```python
from build123d import *

# Parameters (mm, degrees)
F1_DEPTH = 23
F2_W     = 55.3733881378
F2_H     = 29.1305183362
F3_DEPTH = 2


with BuildPart() as f1:
    # F0 (on Front) → F1 (new body)
    with BuildSketch(Plane.XZ):
        with BuildLine():
            Line((58.6916125421, -112.6401221338), (58.6916125421, -83.5096037976))
            ThreePointArc((58.6916125421, -83.5096037976), (63.4212285001, -31.2054716299), (12.2713760607, -19.2981585681))
            Line((12.2713760607, -19.2981585681), (12.2713760607, 27.3598778662))
            Line((12.2713760607, 27.3598778662), (0.550356732, 27.3598778662))
            Line((0.550356732, 27.3598778662), (0.550356732, -28.7071379409))
            ThreePointArc((0.550356732, -28.7071379409), (-8.9441612758, -56.657800803), (3.3182244043, -83.5096037976))
            Line((3.3182244043, -83.5096037976), (3.3182244043, -112.6401221338))
            Line((3.3182244043, -112.6401221338), (58.6916125421, -112.6401221338))
        make_face()
    extrude(amount=F1_DEPTH)

    # F2 (on face) → F3 (cut)
    with BuildSketch(Plane(origin=(0, 0, 0), x_dir=(-1, 0, 0), z_dir=(0, 1, 0))):
        with Locations((-31.0049184732, -98.0748629657)):
            Rectangle(F2_W, F2_H)
    extrude(amount=-F3_DEPTH, mode=Mode.SUBTRACT)


solid = f1.part
```
Model file for the job. Use its own axes, mm. A direction names the side the tool comes from. Coordinates: 2 decimals unless noted, no trailing zeros. Loops run counter-clockwise (first coordinate to the right, second up) from the corner with the lowest first, then second, coordinate; pieces in that order, holes last. Notation, with made-up numbers: (32, -28.5) - (67, -28.5) arc R13 cw to (67, -5.5) - close; hole circle Ø11 at (34.5, 79). An arc over 180 degrees is marked (long way). Answer as a JSON object with one key per item and string values. Group by question number.
(1) Flat gauge pins, fed straight in: pin 1 (1 mm diameter, centred on x = 27.5, y = -0.5, fed in from -Z); pin 2 (12 mm diameter, centred on y = -4.5, z = -74, fed in from +X); pin 3 (8 mm diameter, centred on x = 46, y = -6, fed in from +Z). Where does each tip first touch, or does it go through?
(2) Tool access for faces 1 (the face through (58.692, -12, -98)), 2 (the face through (0.55, -11, 0)), 3 (the face through (31, -2, -98)), 4 (the face through (6, -11, 27.36)), 5 (the face through (3.318, -12, -98)): list every direction of +Z, -Z, +X, -X, +Y, -Y with a clear straight run to the whole face (end or side of a thin tool).
(3) Probe line 1 along X through (y, z) = (-10, -97.5); line 2 along X through (y, z) = (-9.25, -7); line 3 along Y through (x, z) = (6, -95). List the from-to ranges inside material, lowest first.
(4) Cut at D-D (x = 22.5). Give the cut face in (y, z).
(5) Cut at A-A (y = -15.75). Give the cut face in (x, z).
(6) Cut at B-B (x = 8). Give the cut face in (y, z), then the cut area to 3 significant figures.
(7) Cut at C-C (z = -88). Give the cut face in (x, y).
Geometry says:
{
 "1": {"pin 1": "stops at z = -83.51", "pin 2": "stops at x = 68.71", "pin 3": "stops at z = -16.18"},
 "2": {"face 1": "-Z, +X, +Y, -Y", "face 2": "+Z, -X, +Y, -Y", "face 3": "-Z, +X, -X, +Y", "face 4": "+Z, +X, -X, +Y, -Y", "face 5": "-Z, -X, +Y, -Y"},
 "3": {"line 1": "x = 3.32 to 58.69", "line 2": "x = 0.55 to 12.27", "line 3": "y = -23 to -2"},
 "4": {"outline": "(-23, -112.64) - (-2, -112.64) - (-2, -83.51) - (0, -83.51) - (0, -15.55) - (-23, -15.55) - close"},
 "5": {"outline": "(0.55, -28.71) arc R40 ccw to (3.32, -83.51) - (3.32, -112.64) - (58.69, -112.64) - (58.69, -83.51) arc R40 ccw to (12.27, -19.3) - (12.27, 27.36) - (0.55, 27.36) - close"},
 "6": {"outline": "(-23, -112.64) - (-2, -112.64) - (-2, -83.51) - (0, -83.51) - (0, 27.36) - (-23, 27.36) - close", "area": "3,160 mm^2"},
 "7": {"outline": "(3.32, -23) - (58.69, -23) - (58.69, -2) - (3.32, -2) - close"}
}
